Check sheet for the modelled part. Datum: model origin and axes. Units: mm. Face numbers are marked on the shaded views. A direction names the side the tool comes from. Round coordinates to 2 decimals unless told otherwise and drop trailing zeros. Order: outer loops, then holes, each group sorted by start corner. A loop starts at its lowest first (then second) coordinate and runs counter-clockwise, first axis right, second up.
(1) Thickness scan on probe 1 along Z at (x, y) = (-3, 19); probe 2 along X at (y, z) = (4.5, 12.25); probe 3 along Y at (x, z) = (16.5, 0.75). Record the ranges inside material, lowest first.
(2) Depth check by flat-ended pin: pin 1 (2 mm diameter, centred on x = 19.5, y = -15, fed in from +Z); pin 2 (8 mm diameter, centred on y = 10, z = 12, fed in from +X); pin 3 (1 mm diameter, centred on y = -8.5, z = 2.5, fed in from +X). Enter the tip coordinate at first touch or a pass-through.
(3) Mould release check, pull along Y, two halves, no side actions. Record for the marked faces 3, 4 and 5: released by +Y, released by -Y, zero draft, split by the parting line, or undercut.
(4) Sectioned sample at D-D, the plane z = 4.5. Enter the section's corners in (x, y).
(5) Sectioned sample at A-A, the plane z = 13. Enter the section's corners in (x, y), and give its area (3 significant figures).
(6) Tool access check on the marked faces 1 and 2. Record the directions out of +Z, -Z, +X, -X, +Y, -Y that give a thin tool (end or side, any length) a straight path to the whole face; none if there is none.
(7) Sectioned sample at B-B, the plane x = 6. Enter the section's corners in (y, z).
Autodesk Inventor part; units mm, degrees
ref_plane "YZ Plane" through (0, 0, 0) normal (1, 0, 0) x (0, 1, 0)
ref_plane "XZ Plane" through (0, 0, 0) normal (0, 1, 0) x (-1, 0, 0)
ref_plane "XY Plane" through (0, 0, 0) normal (0, 0, 1) x (1, 0, 0)
sketch "Boceto1" plane through (0, 0, 0) normal (0, 0, 1) x (1, 0, 0)
  circle A0 centre (0, 0) radius 25
  dimension "d0" = 50
extrude "Extrusión1" add sketch "Boceto1" along normal blind 10
sketch "Boceto3" plane through (0, 0, 10) normal (0, 0, 1) x (1, 0, 0)
  circle A0 centre (-6, -6) radius 2.5
  line L0 (0, 35) -> (0, -35)
  line L1 (-35, 0) -> (35, 0)
  circle A1 centre (6, -6) radius 2.5
  circle A2 centre (6, 6) radius 2.5
  circle A3 centre (-6, 6) radius 2.5
  line L2 (-18, -22) -> (18, -22)
  line L3 (18, -22) -> (18, 22)
  line L4 (18, 22) -> (-18, 22)
  line L5 (-18, 22) -> (-18, -22)
  point P0 (0, 0)
  dimension "d3" = 5
  dimension "d4" = 6
  dimension "d5" = 6
  dimension "d8" = 360
  dimension "d12" = 44
  dimension "d13" = 36
  dimension "d14" = 18
  dimension "d16" = 22
extrude "Extrusión2" add sketch "Boceto3" along normal blind 4 contours A0 | A1 | A2 | A3
properties part number "BaseH"
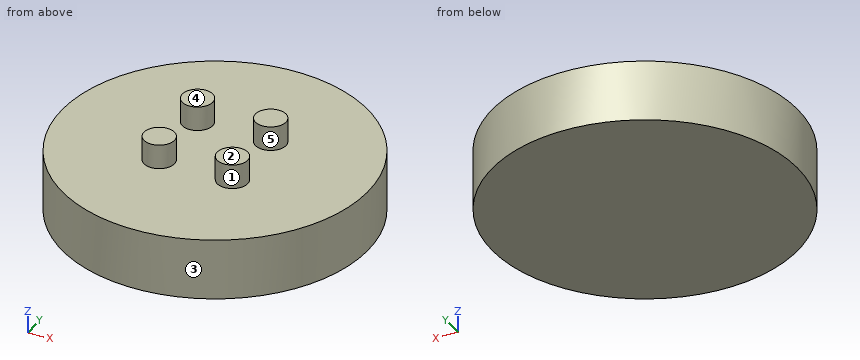
Derived:
1. probe 1: z = 0 to 10
1. probe 2: x = -8 to -4, 4 to 8
1. probe 3: y = -18.78 to 18.78
2. pin 1: stops at z = 10
2. pin 2: stops at x = 24.13
2. pin 3: stops at x = 23.69
3. face 3: split by the parting line
3. face 4: zero draft
3. face 5: undercut
4. outline: circle Ø50 at (0, 0)
5. outline: circle Ø5 at (-6, -6); circle Ø5 at (-6, 6); circle Ø5 at (6, -6); circle Ø5 at (6, 6)
5. area: 78.5 mm2
6. face 1: +Z
6. face 2: +Z, +X, -X, +Y, -Y
7. outline: (-24.27, 0) - (24.27, 0) - (24.27, 10) - (8.5, 10) - (8.5, 14) - (3.5, 14) - (3.5, 10) - (-3.5, 10) - (-3.5, 14) - (-8.5, 14) - (-8.5, 10) - (-24.27, 10) - close
